Could you check a few things on this drawing? It's one solid part, dimensions in mm from its lowest x, y, z. Give positions to 0.01 mm unless a question says otherwise; leave off trailing zeros. Order: outer loops, then holes, each group sorted by start corner. A loop starts at its lowest first (then second) coordinate and runs counter-clockwise, first axis right, second up. Notation, with made-up numbers: (82.5, 66.5) -> (116.5, 66.5) arc R27 ccw to (116.5, 103.5) -> close; hole circle Ø8 at (69, -1.5). An arc over 180 degrees is marked (long way). Write each question's results on one line, items separated by ' | '.
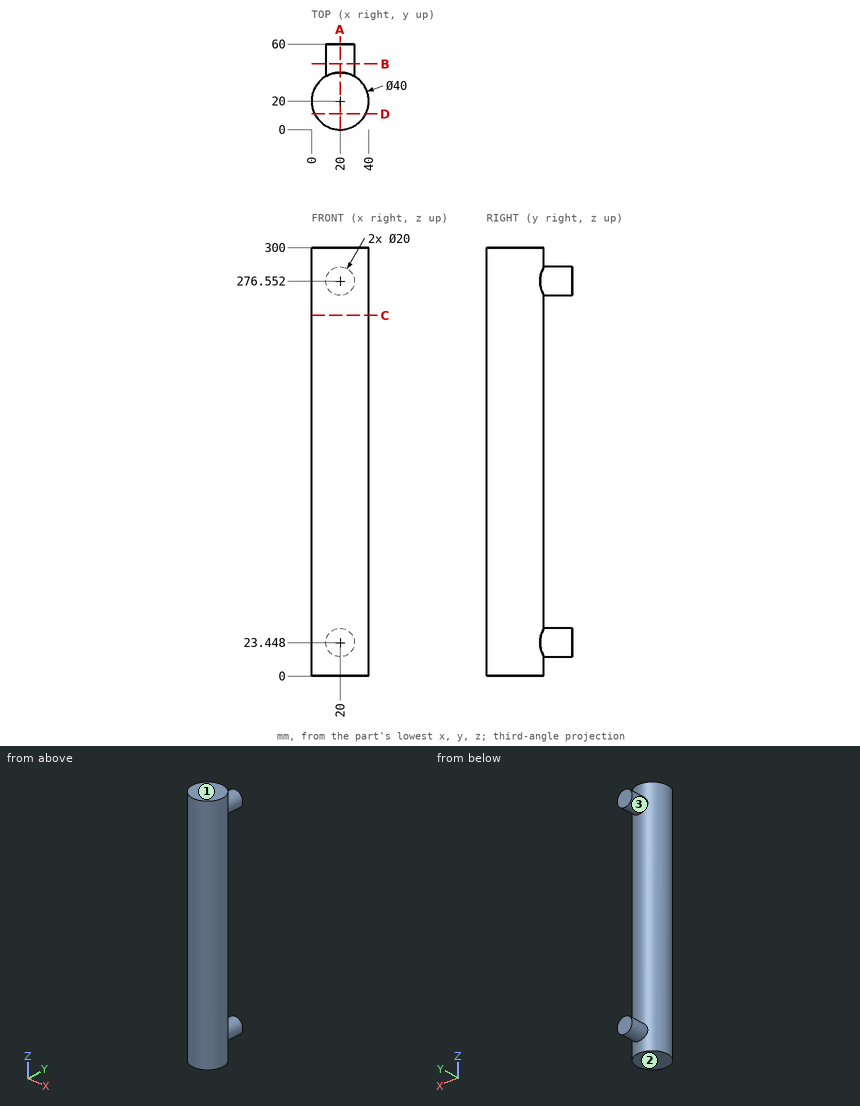
Q1. Suppose I cut it at A-A on x = 20. Please give me the cut outline in (y, z), and give its area (3 significant figures).
Here are the results:
outline: (0, 0) -> (40, 0) -> (40, 13.45) -> (60, 13.45) -> (60, 33.45) -> (40, 33.45) -> (40, 266.55) -> (60, 266.55) -> (60, 286.55) -> (40, 286.55) -> (40, 300) -> (0, 300) -> close | area: 12,800 mm²
Q2. Suppose I cut it at C-C on z = 252.5. Please give me the cut outline in (x, y).
Here are the results:
outline: circle Ø40 at (20, 20)
Q3. I'm going to push flat-ended pins straight in: pin 1 Ø8 at (x, y) = (31, 51.5) entering from +Z; pin 2 Ø1.5 at (x, z) = (22.5, 69.5) entering from +Y; pin 3 Ø4 at (y, z) = (24, 89.5) entering from -X. Where does each tip first touch, or does it pass through?
Here are the results:
pin 1: stops at z = 283.69 | pin 2: stops at y = 39.92 | pin 3: stops at x = 0.1
Q4. Suppose I cut it at D-D on y = 11. Please give me the cut outline in (x, z).
Here are the results:
outline: (2.14, 0) -> (37.86, 0) -> (37.86, 300) -> (2.14, 300) -> close
Q5. Suppose I cut it at B-B on y = 46. Please give me the cut outline in (x, z), and give its area (3 significant figures).
Here are the results:
outline: circle Ø20 at (20, 23.45); circle Ø20 at (20, 276.55) | area: 628 mm²
Q6. I need wall thicknesses on line 1 along Y through (x, z) = (18.5, 182.5); line 2 along Z through (x, y) = (29, 41) (1 decimal); line 3 along X through (y, z) = (42.5, 283) (1 decimal). Which ranges of each line are inside material? Lowest first, please.
Here are the results:
line 1: y = 0.06 to 39.94 | line 2: z = 19.1 to 27.8, 272.2 to 280.9 | line 3: x = 12.4 to 27.6
Q7. Thinking about a two-plate mould opening in Z: for the marked faces 1, 2 and 3, which applies, +Z half, -Z half, draft (parallel to the pull), parting line (faces both ways), or undercut?
Here are the results:
face 1: +Z half | face 2: -Z half | face 3: undercut
